```python
from build123d import *

# Parameters (mm, degrees)
SKETCH2_R             = 5.07
CUT_EXTRUDE1_DEPTH    = 33.787192622
CHAMFER1_SIZE         = 0.5
FILLET1_R             = 0.2
SKETCH3_R             = 4.5
CUT_EXTRUDE2_DEPTH    = 11
M5_TAPPED_HOLE1_D     = 4.2
M5_TAPPED_HOLE1_DEPTH = 10
M5_TAPPED_HOLE1_TIP   = 1.2618073


# Read off the part's stored shape, not the designer's step: Draft1
with BuildPart() as part:
    # Sketch1 → Revolve1 (revolve)
    with BuildSketch(Plane.XY, mode=Mode.PRIVATE) as revolve1_sk:
        Polygon((0, 0), (15, 0), (15, -15), (7.5, -15), (7.5, -25), (0, -25), align=None)
    revolve(revolve1_sk.sketch.rotate(Axis((0, -30, 0), (0, 1, 0)), 90), axis=Axis((0, -30, 0), (0, 1, 0)))

    # Sketch2 → Cut-Extrude1 (cut, through all)
    with BuildSketch(Plane(origin=(0, 0, 0), x_dir=(1, 0, 0), z_dir=(0, 1, 0))):
        with Locations(Location((0, 0, 0), (0, 0, 180))):
            Circle(SKETCH2_R)
    extrude(amount=-CUT_EXTRUDE1_DEPTH, mode=Mode.SUBTRACT)

    # Chamfer1
    chamfer1_edges = [part.edges().sort_by_distance(p)[0] for p in [
        (0, -25, 7.5),
        (0, -15, 15),
        (0, 0, 15),
    ]]
    chamfer(chamfer1_edges, length=CHAMFER1_SIZE)

    # Fillet1
    fillet1_edges = [part.edges().sort_by_distance(p)[0] for p in [
        (0, -15, 7.5),
    ]]
    fillet(fillet1_edges, radius=FILLET1_R)

    # Draft1 outline → Draft1 (revolve, cut)
    with BuildSketch(Plane.XY):
        Polygon((5.450520415, -25), (5.07, -3.2), (5.07, -25), align=None)
    revolve(axis=Axis((0, 0, 0), (0, 1, 0)), mode=Mode.SUBTRACT)

    # Sketch3 → Cut-Extrude2 (cut)
    with BuildSketch(Plane(origin=(0, 0, 0), x_dir=(1, 0, 0), z_dir=(0, 1, 0))):
        with Locations((-18, 0)):
            Circle(SKETCH3_R)
    cut_extrude2 = extrude(amount=-CUT_EXTRUDE2_DEPTH, mode=Mode.SUBTRACT)

    # Mirror1: Cut-Extrude2 across plane
    add(cut_extrude2.mirror(Plane(origin=(0, 0, 0), x_dir=(0, 0, 1), z_dir=(1, 0, 0))), mode=Mode.SUBTRACT)

    # M5 Tapped Hole1
    with Locations(Plane(origin=(0, 0, 0), x_dir=(1, 0, 0), z_dir=(0, 1, 0))):
        with Locations((0, 11), (0, -11)):
            Hole(M5_TAPPED_HOLE1_D / 2, depth=M5_TAPPED_HOLE1_DEPTH)
            with Locations((0, 0, -(M5_TAPPED_HOLE1_DEPTH + M5_TAPPED_HOLE1_TIP / 2))):  # 118° drill point
                Cone(0, M5_TAPPED_HOLE1_D / 2, M5_TAPPED_HOLE1_TIP, mode=Mode.SUBTRACT)


solid = part.part
```
Verification items for the finished model (mm, model axes). A direction names the side the tool comes from. Round coordinates to 2 decimals unless told otherwise and drop trailing zeros. Write each loop counter-clockwise with the first axis right and the second up, starting at its lowest first coordinate (ties: lowest second). Pieces come first, ordered by that corner, then holes.
1. Draft check along X on faces 4 (the conical face through (-0.047, -11.043, -11.362)), 5 (the cylindrical face through (14.643, -7.598, 3.252)), 6 (the flat face through (6, -15, -6)). Enter one of: +X half, -X half, draft (parallel to the pull), parting line (faces both ways), or undercut.
2. Section check A-A on y = -17.25. Enter the section's corners in (x, z).
3. Gauge pin test, flat ends, axial feed: P1, Ø8, axis at y = -4, z = 11, coming from the +X side; P2, Ø6, axis at x = -5.5, y = -12.5, coming from the +Z side; P3, Ø8, axis at x = 3, z = -4.5, coming from the +Y side; P4, Ø1, axis at y = -6, z = 0, coming from the -X side. Record the tip position at first contact, or that the pin passes through.
4. Access from +Z, -Z, +X, -X, +Y, -Y to the whole of each face (thin tool, end or side, straight path). Record for faces 1 (the flat face through (14, -11, 0)), 2 (the cylindrical face through (-13.5, -5.4, 0)), 3 (the cylindrical face through (0.273, -5.07, 8.918)).
5. Scan lines: L1, parallel to Z at x = 0.25, y = -7.25; L2, parallel to Y at x = 7, z = -6; L3, parallel to X at y = -7.25, z = 11. Record each from-to range of solid material in increasing order.
Answer:
1. face 4: undercut
1. face 5: parting line
1. face 6: draft
2. outline: circle Ø15 at (0, 0); hole circle Ø10.63 at (0, 0)
3. P1: stops at x = 13.27
3. P2: stops at z = 14.79
3. P3: stops at y = 0
3. P4: stops at x = -13.53
4. face 1: +X, +Y
4. face 2: -X, +Y
4. face 3: +Y
5. L1: z = -15 to -13.09, -8.91 to -5.13, 5.13 to 8.91, 13.09 to 15
5. L2: y = -15 to 0
5. L3: x = -10.2 to -2.1, 2.1 to 10.2
